For this review, take the finished solid that the model builds, in its own axes (mm). Face numbers are marked on the shaded views. A direction names the side the tool comes from. Coordinates: 2 decimals unless noted, no trailing zeros. Order: outer loops, then holes, each group sorted by start corner. A loop starts at its lowest first (then second) coordinate and runs counter-clockwise, first axis right, second up. Notation, with made-up numbers: M 9.25,59 L 47.25,59 A26 ccw 47.25,79 Z; hole C -9.75,-26.5 d2. An arc over 180 degrees is marked long. Use CSV: the item, a comma, the result in double quotes.
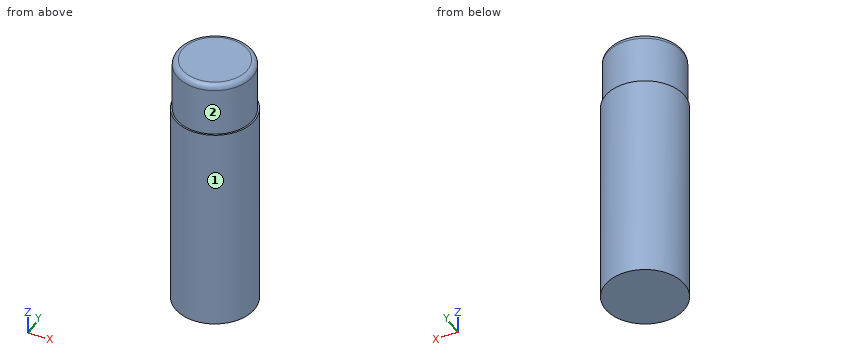
```python
from build123d import *

# Parameters (mm, degrees)
SKIZZE1_R                       = 3.5
AUFSATZ_LINEAR_AUSTRAGEN1_DEPTH = 24.5
VERRUNDUNG1_R                   = 0.5
SKIZZE2_R                       = 3.65
AUFSATZ_LINEAR_AUSTRAGEN2_DEPTH = 19.5


with BuildPart() as part:
    # Skizze1 → Aufsatz-Linear austragen1 (new body)
    with BuildSketch(Plane.XY):
        Circle(SKIZZE1_R)
    extrude(amount=AUFSATZ_LINEAR_AUSTRAGEN1_DEPTH)

    # Verrundung1
    verrundung1_edges = [part.edges().sort_by_distance(p)[0] for p in [
        (-3.5, 0, 24.5),
    ]]
    fillet(verrundung1_edges, radius=VERRUNDUNG1_R)

    # Skizze2 → Aufsatz-Linear austragen2 (add)
    with BuildSketch(Plane(origin=(0, 0, 0), x_dir=(-1, 0, 0), z_dir=(0, 0, -1))):
        Circle(SKIZZE2_R)
    extrude(amount=-AUFSATZ_LINEAR_AUSTRAGEN2_DEPTH)


solid = part.part
```
Item 1: For the marked faces 1 and 2, list the 3-axis set-ups (+Z, -Z, +X, -X, +Y, -Y) from which the entire face can be reached by the end or side of a thin tool; tool diameter is ignored.
Solutions:
face 1,"+Z, -Z"
face 2,"+Z"
Item 2: To check wall thickness, follow line 1 along X through (y, z) = (-3, 14.5); line 2 along Y through (x, z) = (2, 19.75); line 3 along Z through (x, y) = (2.25, -2.5). State the ranges of each line that lie inside material, in increasing order. Write a range as [from, to].
Solutions:
line 1,"[-2.08, 2.08]"
line 2,"[-2.87, 2.87]"
line 3,"[0, 24.34]"
Item 3: Clearance check with flat-ended pins moving along their axes: pin 1 Ø3 at (y, z) = (3, 13) entering from -X; pin 2 Ø3 at (y, z) = (-1.5, 12.5) entering from +X; pin 3 Ø1 at (x, z) = (-1.5, 16) entering from +Y. State where each tip first meets the part, or that it passes through.
Solutions:
pin 1,"x = -3.33"
pin 2,"x = 3.65"
pin 3,"y = 3.51"
Item 4: Add section A-A on z = 14. State the section outline as (x, y) points, and give its area (3 significant figures).
Solutions:
outline,"C 0,0 d7.3"
area,"41.9 mm^2"
